from build123d import *

# Parameters (mm, degrees)
SKETCH1_W               = 50
SKETCH1_H               = 10
BOSS_EXTRUDE1_DEPTH     = 6
SKETCH2_R               = 2.85
SKETCH2_R_2             = 1.5
CUT_EXTRUDE1_DEPTH      = 4
SKETCH3_R               = 1.5
CUT_EXTRUDE2_DEPTH      = 4
FILLET1_R               = 1.5
SKETCH6_W               = 23.5
SKETCH6_H               = 7
BOSS_EXTRUDE3_DEPTH     = 3.01
CUT_EXTRUDE4_DEPTH      = 27.191601707
CUT_EXTRUDE4_DEPTH_BACK = 27.191601707
SKETCH7_R               = 1.75
SKETCH8_R               = 1.5
CUT_EXTRUDE5_DEPTH      = 10


with BuildPart() as part:
    # Sketch1 → Boss-Extrude1 (new body)
    with BuildSketch(Plane(origin=(0, 0, 0), x_dir=(1, 0, 0), z_dir=(0, 1, 0))):
        Rectangle(SKETCH1_W, SKETCH1_H)
    extrude(amount=BOSS_EXTRUDE1_DEPTH)

    # Sketch2 → Cut-Extrude1 (cut)
    with BuildSketch(Plane(origin=(0, 6, 0), x_dir=(1, 0, 0), z_dir=(0, 1, 0))):
        with Locations(Location((-19.15, 0, 0), (0, 0, 270))):
            Circle(SKETCH2_R)
        with Locations(Location((16.85, 0, 0), (0, 0, 270))):
            Circle(SKETCH2_R_2)
    extrude(amount=-CUT_EXTRUDE1_DEPTH, mode=Mode.SUBTRACT)

    # Sketch3 → Cut-Extrude2 (cut)
    with BuildSketch(Plane(origin=(0, 2, 0), x_dir=(1, 0, 0), z_dir=(0, 1, 0))):
        with Locations(Location((16.85, 0, 0), (0, 0, 270))):
            Circle(SKETCH3_R)
    extrude(amount=-CUT_EXTRUDE2_DEPTH, mode=Mode.SUBTRACT)

    # Fillet1
    fillet1_edges = [part.edges().sort_by_distance(p)[0] for p in [
        (-25, 6, 0),
        (0, 6, 5),
        (25, 6, 0),
        (0, 0, 5),
        (-25, 0, 0),
        (0, 0, -5),
        (25, 0, 0),
        (25, 3, 5),
        (-25, 3, 5),
        (-25, 3, -5),
        (25, 3, -5),
        (0, 6, -5),
    ]]
    fillet(fillet1_edges, radius=FILLET1_R)

    # Sketch6 → Boss-Extrude3 (add)
    with BuildSketch(Plane.XZ):
        with Locations((11.75, 0)):
            Rectangle(SKETCH6_W, SKETCH6_H)
    extrude(amount=BOSS_EXTRUDE3_DEPTH)

    # Sketch7 → Cut-Extrude4 (cut, two sides: drawn at the far end of the back side and taken through both)
    with BuildSketch(Plane(origin=(0, 0, 0), x_dir=(1, 0, 0), z_dir=(0, 1, 0)).offset(-CUT_EXTRUDE4_DEPTH_BACK)):
        with Locations(Location((16.85, 0, 0), (0, 0, 270))):
            Circle(SKETCH7_R)
    extrude(amount=CUT_EXTRUDE4_DEPTH + CUT_EXTRUDE4_DEPTH_BACK, mode=Mode.SUBTRACT)

    # Sketch8 → Cut-Extrude5 (cut)
    with BuildSketch(Plane(origin=(0, 2, 0), x_dir=(1, 0, 0), z_dir=(0, 1, 0))):
        with Locations(Location((-19.15, 0, 0), (0, 0, 270))):
            Circle(SKETCH8_R)
    extrude(amount=-CUT_EXTRUDE5_DEPTH, mode=Mode.SUBTRACT)


solid = part.part
Design review of the part built by this model. Coordinates are the model's own, in mm. A direction names the side the tool comes from. Round coordinates to 2 decimals unless told otherwise and drop trailing zeros. Loops run counter-clockwise (first coordinate to the right, second up) from the corner with the lowest first, then second, coordinate; pieces in that order, holes last. Notation, with made-up numbers: (62.25, 7) - (95.25, 7) arc R18 ccw to (95.25, 11) - close; hole circle Ø1 at (27, 50). An arc over 180 degrees is marked (long way). One line per question, with ' | ' between items.
1. We need section A-A, the plane x = 16.85. State the section outline as (y, z) points, and give its area (3 significant figures).
Results are:
outline: (-3.01, -3.5) - (0, -3.5) arc R1.5 ccw to (1.5, -5) - (4.5, -5) arc R1.5 ccw to (6, -3.5) - (6, -1.75) - (-3.01, -1.75) - close; (-3.01, 1.75) - (6, 1.75) - (6, 3.5) arc R1.5 ccw to (4.5, 5) - (1.5, 5) arc R1.5 ccw to (0, 3.5) - (-3.01, 3.5) - close | area: 47.6 mm²
2. We need section C-C, the plane y = -0.5. State the section outline as (x, z) points.
Results are:
outline: (0, -3.5) - (23.5, -3.5) - (23.5, 3.5) - (0, 3.5) - close; hole circle Ø3.5 at (16.85, 0)
3. For L1, parallel to Z at x = 16.85, y = 3.5; L2, parallel to X at y = 1, z = 0; L3, parallel to X at y = 5, z = -1.5, list the stretches that pass through material, from the lowest coordinate up. Write a range as [from, to].
Results are:
L1: z = [-5, -1.75], [1.75, 5] | L2: x = [-24.91, -20.65], [-17.65, 15.1], [18.6, 24.91] | L3: x = [-24.91, -21.57], [-16.73, 15.95], [17.75, 24.91]
4. Draft analysis for pull direction Z (two halves, no side actions). For faces 1 (the face through (-24.57, 3.02, -4.55)), 2 (the face through (-20.4, 2, 1.2)), 3 (the face through (-12, 0, 0)), 4 (the face through (15.3, 1.43, 0.81)), state which applies: released by +Z, released by -Z, zero draft, split by the parting line, or undercut.
Results are:
face 1: released by -Z | face 2: undercut | face 3: zero draft | face 4: undercut
5. For faces 5 (the face through (24.57, 3.02, -4.55)), 6 (the face through (0, -1, 0)), 7 (the face through (12, -1, -3.5)), 8 (the face through (-21.93, 4.03, -0.62)), 9 (the face through (12, -1, 3.5)), list the 3-axis set-ups (+Z, -Z, +X, -X, +Y, -Y) from which the entire face can be reached by the end or side of a thin tool; tool diameter is ignored.
Results are:
face 5: -Z, +X, +Y, -Y | face 6: +Z, -Z, -X, -Y | face 7: -Z, +X, -X, -Y | face 8: +Y | face 9: +Z, +X, -X, -Y
6. We need section D-D, the plane x = -7.5. State the section outline as (y, z) points.
Results are:
outline: (0, -3.5) arc R1.5 ccw to (1.5, -5) - (4.5, -5) arc R1.5 ccw to (6, -3.5) - (6, 3.5) arc R1.5 ccw to (4.5, 5) - (1.5, 5) arc R1.5 ccw to (0, 3.5) - close
7. Clearance check with flat-ended pins moving along their axes: P1, Ø1.5, axis at x = 10, y = -2, coming from the -Z side; P2, Ø2.5, axis at y = -1.5, z = 1.5, coming from the +X side; P3, Ø0.9, axis at x = 13, y = -1, coming from the +Z side. State where each tip first meets the part, or that it passes through.
Results are:
P1: stops at z = -3.5 | P2: stops at x = 23.5 | P3: stops at z = 3.5
8. We need section B-B, the plane z = 0. State the section outline as (x, y) points.
Results are:
outline: (-25, 1.5) arc R1.5 ccw to (-23.5, 0) - (-20.65, 0) - (-20.65, 2) - (-22, 2) - (-22, 6) - (-23.5, 6) arc R1.5 ccw to (-25, 4.5) - close; (-17.65, 0) - (0, 0) - (0, -3.01) - (15.1, -3.01) - (15.1, 6) - (-16.3, 6) - (-16.3, 2) - (-17.65, 2) - close; (18.6, -3.01) - (23.5, -3.01) - (23.5, 0) arc R1.5 ccw to (25, 1.5) - (25, 4.5) arc R1.5 ccw to (23.5, 6) - (18.6, 6) - close
